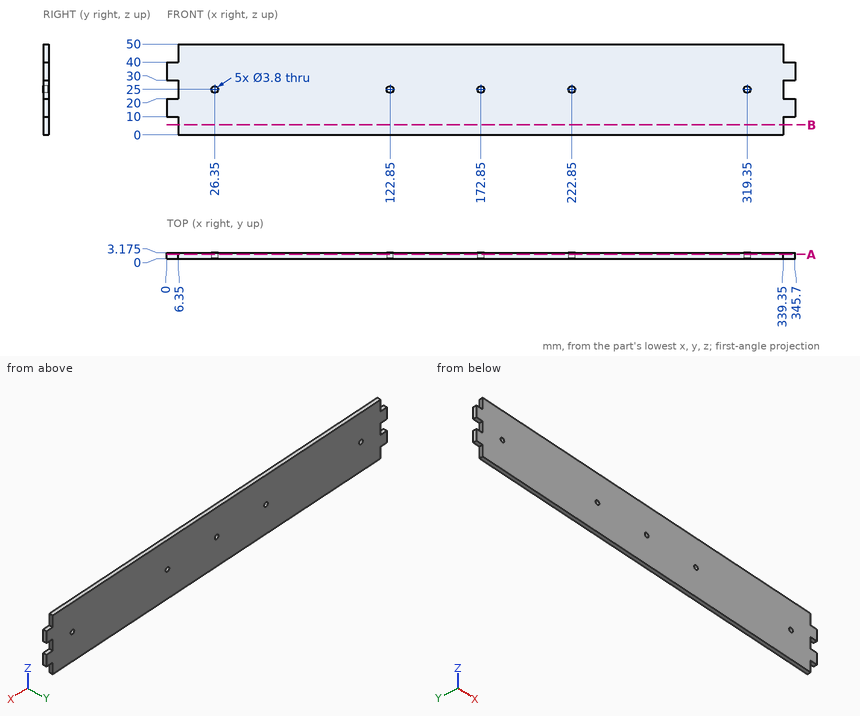
Answer from the drawing. Dimensions are ordinates in mm from the lowest x, y and z of the part. Coordinates: 2 decimals unless noted, no trailing zeros. Loops run counter-clockwise (first coordinate to the right, second up) from the corner with the lowest first, then second, coordinate; pieces in that order, holes last. Notation, with made-up numbers: (83, 32.5) - (87, 32.5) arc R28 ccw to (87, 64.5) - close; hole circle Ø6 at (31, 48). An arc over 180 degrees is marked (long way). Use a Markdown table: item, result.
Item 1: Given pin 1 Ø2.5 at (x, z) = (319.35, 25) entering from +Y; pin 2 Ø1.6 at (x, y) = (342, 1.5) entering from +Z; pin 3 Ø1 at (y, z) = (2, 23.5) entering from +X; pin 4 Ø1.6 at (x, y) = (341, 1.5) entering from -Z, each flat-ended and moving along its own axis, determine where each tip first touches the part or whether it passes through.
Evaluation:
| item | result |
|---|---|
| pin 1 | passes through |
| pin 2 | stops at z = 40 |
| pin 3 | stops at x = 339.35 |
| pin 4 | stops at z = 10 |
Item 2: Find section A-A, the plane y = 2.35. Determine the outline of the cut face in (x, z).
Evaluation:
| item | result |
|---|---|
| outline | (0, 10) - (6.35, 10) - (6.35, 0) - (339.35, 0) - (339.35, 10) - (345.7, 10) - (345.7, 20) - (339.35, 20) - (339.35, 30) - (345.7, 30) - (345.7, 40) - (339.35, 40) - (339.35, 50) - (6.35, 50) - (6.35, 40) - (0, 40) - (0, 30) - (6.35, 30) - (6.35, 20) - (0, 20) - close; hole circle Ø3.8 at (26.35, 25); hole circle Ø3.8 at (122.85, 25); hole circle Ø3.8 at (172.85, 25); hole circle Ø3.8 at (222.85, 25); hole circle Ø3.8 at (319.35, 25) |
Item 3: Find section B-B, the plane z = 5.5. Determine the outline of the cut face in (x, y) (3 decimals), and give its area (3 significant figures).
Evaluation:
| item | result |
|---|---|
| outline | (6.35, 0) - (339.35, 0) - (339.35, 3.175) - (6.35, 3.175) - close |
| area | 1,060 mm2 |
Item 4: Consider probe 1 along X at (y, z) = (0.9, 25); probe 2 along Z at (x, y) = (172.85, 1.05); probe 3 along X at (y, z) = (0.4, 22). Determine where each line is inside the solid, lowest interval first. Write a range as from..to.
Evaluation:
| item | result |
|---|---|
| probe 1 | x = 6.35..24.45, 28.25..120.95, 124.75..170.95, 174.75..220.95, 224.75..317.45, 321.25..339.35 |
| probe 2 | z = 0..23.1, 26.9..50 |
| probe 3 | x = 6.35..339.35 |
